Verification items for the finished model (mm, model axes). Face numbers are marked on the shaded views. A direction names the side the tool comes from. Coordinates: 2 decimals unless noted, no trailing zeros. Order: outer loops, then holes, each group sorted by start corner. A loop starts at its lowest first (then second) coordinate and runs counter-clockwise, first axis right, second up. Notation, with made-up numbers: M -27.5,-18 L -18.5,-18 A6 cw -18.5,-7 Z; hole C -26.5,-40 d2. An arc over 180 degrees is marked long. Return JSON: item names as keys, results as strings.
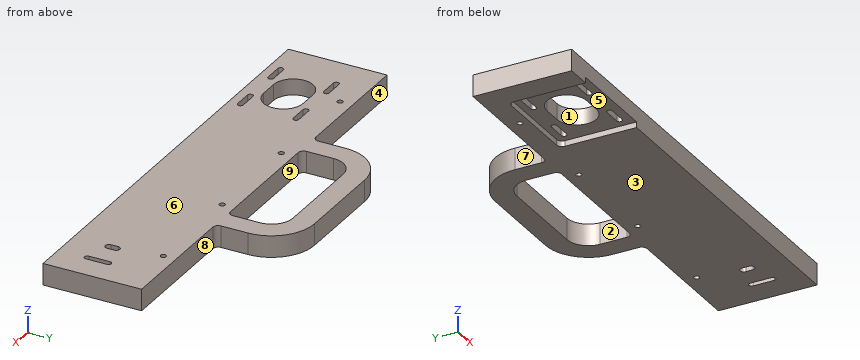
```python
from build123d import *

# Parameters (mm, degrees)
SKIZZE2_R                       = 1.55
SKIZZE2_W                       = 75
SKIZZE2_H                       = 30
AUFSATZ_LINEAR_AUSTRAGEN1_DEPTH = 12
SKIZZE2_3_W                     = 52
SKIZZE2_3_H                     = 43
SCHNITT_LINEAR_AUSTRAGEN1_DEPTH = 3.11
VERRUNDUNG1_R                   = 12
VERRUNDUNG2_R                   = 24
VERRUNDUNG3_R                   = 3
VERRUNDUNG4_R                   = 3


with BuildPart() as part:
    # Skizze2 → Aufsatz-Linear austragen1 (new body)
    with BuildSketch(Plane.XY):
        Polygon((-125, 27.5), (-125, -27.5), (125, -27.5), (125, 27.5), (49.5, 27.5), (49.5, 69.5), (-49.5, 69.5), (-49.5, 27.5), align=None)
        with Locations((-90, 20.5)):
            Circle(SKIZZE2_R, mode=Mode.SUBTRACT)
        with Locations((-30, 20.5)):
            Circle(SKIZZE2_R, mode=Mode.SUBTRACT)
        with BuildLine():
            ThreePointArc((92.175, -3.5), (94.225, -1.45), (96.275, -3.5))
            Line((96.275, -3.5), (96.275, -7.5))
            ThreePointArc((96.275, -7.5), (94.225, -9.55), (92.175, -7.5))
            Line((92.175, -7.5), (92.175, -3.5))
        make_face(mode=Mode.SUBTRACT)
        with BuildLine():
            ThreePointArc((107.675, 0.45), (109.225, 2), (110.775, 0.45))
            Line((110.775, 0.45), (110.775, -11.45))
            ThreePointArc((110.775, -11.45), (109.225, -13), (107.675, -11.45))
            Line((107.675, -11.45), (107.675, 0.45))
        make_face(mode=Mode.SUBTRACT)
        with Locations((30, 20.5)):
            Circle(SKIZZE2_R, mode=Mode.SUBTRACT)
        with Locations((90, 20.5)):
            Circle(SKIZZE2_R, mode=Mode.SUBTRACT)
        with Locations((0, 42.5)):
            Rectangle(SKIZZE2_W, SKIZZE2_H, mode=Mode.SUBTRACT)
        with BuildLine():
            Line((-74.275, 11.55), (-64.275, 11.55))
            ThreePointArc((-64.275, 11.55), (-62.725, 10), (-64.275, 8.45))
            Line((-64.275, 8.45), (-74.275, 8.45))
            ThreePointArc((-74.275, 8.45), (-75.825, 10), (-74.275, 11.55))
        make_face(mode=Mode.SUBTRACT)
        with BuildLine():
            ThreePointArc((-105.275, -22.55), (-106.825, -21), (-105.275, -19.45))
            Line((-105.275, -19.45), (-95.275, -19.45))
            ThreePointArc((-95.275, -19.45), (-93.725, -21), (-95.275, -22.55))
            Line((-95.275, -22.55), (-105.275, -22.55))
        make_face(mode=Mode.SUBTRACT)
        with BuildLine():
            ThreePointArc((-64.275, -19.45), (-62.725, -21), (-64.275, -22.55))
            Line((-64.275, -22.55), (-74.275, -22.55))
            ThreePointArc((-74.275, -22.55), (-75.825, -21), (-74.275, -19.45))
            Line((-74.275, -19.45), (-64.275, -19.45))
        make_face(mode=Mode.SUBTRACT)
        with BuildLine():
            ThreePointArc((-79.775, 5.5), (-68.775, -5.5), (-79.775, -16.5))
            Line((-79.775, -16.5), (-89.775, -16.5))
            ThreePointArc((-89.775, -16.5), (-100.775, -5.5), (-89.775, 5.5))
            Line((-89.775, 5.5), (-79.775, 5.5))
        make_face(mode=Mode.SUBTRACT)
        with BuildLine():
            ThreePointArc((-105.275, 8.45), (-106.825, 10), (-105.275, 11.55))
            Line((-105.275, 11.55), (-95.275, 11.55))
            ThreePointArc((-95.275, 11.55), (-93.725, 10), (-95.275, 8.45))
            Line((-95.275, 8.45), (-105.275, 8.45))
        make_face(mode=Mode.SUBTRACT)
    extrude(amount=AUFSATZ_LINEAR_AUSTRAGEN1_DEPTH)

    # Skizze2_3 → Schnitt-Linear austragen1 (cut)
    with BuildSketch(Plane.XY):
        with Locations((-84.775, -6)):
            Rectangle(SKIZZE2_3_W, SKIZZE2_3_H)
        with BuildLine():
            ThreePointArc((-89.775, 5.5), (-100.775, -5.5), (-89.775, -16.5))
            Line((-89.775, -16.5), (-79.775, -16.5))
            ThreePointArc((-79.775, -16.5), (-68.775, -5.5), (-79.775, 5.5))
            Line((-79.775, 5.5), (-89.775, 5.5))
        make_face(mode=Mode.SUBTRACT)
        with BuildLine():
            ThreePointArc((-74.275, -19.45), (-75.825, -21), (-74.275, -22.55))
            Line((-74.275, -22.55), (-64.275, -22.55))
            ThreePointArc((-64.275, -22.55), (-62.725, -21), (-64.275, -19.45))
            Line((-64.275, -19.45), (-74.275, -19.45))
        make_face(mode=Mode.SUBTRACT)
        with BuildLine():
            ThreePointArc((-95.275, -22.55), (-93.725, -21), (-95.275, -19.45))
            Line((-95.275, -19.45), (-105.275, -19.45))
            ThreePointArc((-105.275, -19.45), (-106.825, -21), (-105.275, -22.55))
            Line((-105.275, -22.55), (-95.275, -22.55))
        make_face(mode=Mode.SUBTRACT)
        with BuildLine():
            ThreePointArc((-95.275, 8.45), (-93.725, 10), (-95.275, 11.55))
            Line((-95.275, 11.55), (-105.275, 11.55))
            ThreePointArc((-105.275, 11.55), (-106.825, 10), (-105.275, 8.45))
            Line((-105.275, 8.45), (-95.275, 8.45))
        make_face(mode=Mode.SUBTRACT)
        with BuildLine():
            ThreePointArc((-74.275, 11.55), (-75.825, 10), (-74.275, 8.45))
            Line((-74.275, 8.45), (-64.275, 8.45))
            ThreePointArc((-64.275, 8.45), (-62.725, 10), (-64.275, 11.55))
            Line((-64.275, 11.55), (-74.275, 11.55))
        make_face(mode=Mode.SUBTRACT)
    extrude(amount=SCHNITT_LINEAR_AUSTRAGEN1_DEPTH, mode=Mode.SUBTRACT)

    # Verrundung1
    verrundung1_edges = [part.edges().sort_by_distance(p)[0] for p in [
        (37.5, 57.5, 6),
        (-37.5, 57.5, 6),
    ]]
    fillet(verrundung1_edges, radius=VERRUNDUNG1_R)

    # Verrundung2
    verrundung2_edges = [part.edges().sort_by_distance(p)[0] for p in [
        (-49.5, 69.5, 6),
        (49.5, 69.5, 6),
    ]]
    fillet(verrundung2_edges, radius=VERRUNDUNG2_R)

    # Verrundung3
    verrundung3_edges = [part.edges().sort_by_distance(p)[0] for p in [
        (-37.5, 27.5, 6),
        (37.5, 27.5, 6),
        (-49.5, 27.5, 6),
        (49.5, 27.5, 6),
    ]]
    fillet(verrundung3_edges, radius=VERRUNDUNG3_R)

    # Verrundung4
    verrundung4_edges = [part.edges().sort_by_distance(p)[0] for p in [
        (-58.775, 15.5, 1.555),
        (-110.775, 15.5, 1.555),
    ]]
    fillet(verrundung4_edges, radius=VERRUNDUNG4_R)


solid = part.part
```
Q1. Cross-section at A-A, the plane x = 18. Record the boundary of the cut face in (y, z).
Values:
{"outline": "M -27.5,0 L 27.5,0 L 27.5,12 L -27.5,12 Z; M 57.5,0 L 69.5,0 L 69.5,12 L 57.5,12 Z"}
Q2. Cross-section at C-C, the plane z = 6.5. State how many separate pieces and enclosed holes the cut face has, and give its area (3 significant figures).
Values:
{"separate pieces": "1", "enclosed holes": "12", "area": "14,600 mm^2"}
Q3. Tool access check on the marked faces 5, 6, 7, 8 and 9. Record the directions out of +Z, -Z, +X, -X, +Y, -Y that give a thin tool (end or side, any length) a straight path to the whole face; none if there is none.
Values:
{"face 5": "-Z, -Y", "face 6": "+Z, +X, -X, +Y, -Y", "face 7": "+Z, -Z, -X, +Y", "face 8": "+Z, -Z, +X, +Y", "face 9": "+Z, -Z"}
Q4. Go/stop test with flat-tipped pins: pin 1 (3 mm diameter, centred on x = -90.5, z = 1.5, fed in from -Y); pin 2 (21.5 mm diameter, centred on x = -84.5, y = -4, fed in from -Z); pin 3 (2.5 mm diameter, centred on x = -70, z = 6, fed in from +Y). Record where each tip stops, or that it passes through.
Values:
{"pin 1": "y = 15.5", "pin 2": "z = 3.11", "pin 3": "y = 27.5"}
Q5. Material ranges on line 1 along Y through (x, z) = (-102, 6); line 2 along Y through (x, z) = (-90, 4.5); line 3 along X through (y, z) = (41, 8), recorded low to high.
Values:
{"line 1": "-27.5 to -22.55, -19.45 to 8.45, 11.55 to 27.5", "line 2": "-27.5 to -16.5, 5.5 to 18.95, 22.05 to 27.5", "line 3": "-49.5 to -37.5, 37.5 to 49.5"}
Q6. Draft check along Y on the marked faces 1, 2, 3 and 4. Enter one of: pulls with the +Y half, pulls with the -Y half, needs draft (parallel to the pull), parting line crosses it, or undercut.
Values:
{"face 1": "undercut", "face 2": "undercut", "face 3": "needs draft", "face 4": "pulls with the +Y half"}
Q7. Cross-section at B-B, the plane y = 33. Record the boundary of the cut face in (x, z), and give its area (3 significant figures).
Values:
{"outline": "M -49.5,0 L -37.5,0 L -37.5,12 L -49.5,12 Z; M 37.5,0 L 49.5,0 L 49.5,12 L 37.5,12 Z", "area": "288 mm^2"}
Q8. Cross-section at D-D, the plane x = 100. Record the boundary of the cut face in (y, z).
Values:
{"outline": "M -27.5,0 L 27.5,0 L 27.5,12 L -27.5,12 Z"}
